Read the model definition and answer for the solid it produces. Units are mm, in the model's axes. Face numbers are marked on the shaded views. A direction names the side the tool comes from. Give positions to 0.01 mm unless a question says otherwise; leave off trailing zeros. Order: outer loops, then holes, each group sorted by start corner. A loop starts at its lowest first (then second) coordinate and runs counter-clockwise, first axis right, second up. Notation, with made-up numbers: (88, -7) - (144, -7) arc R13 ccw to (144, 17) - close; hole circle Ø1 at (3, 22.5). An arc over 180 degrees is marked (long way). One line per item, written item: value. Start each with the question number.
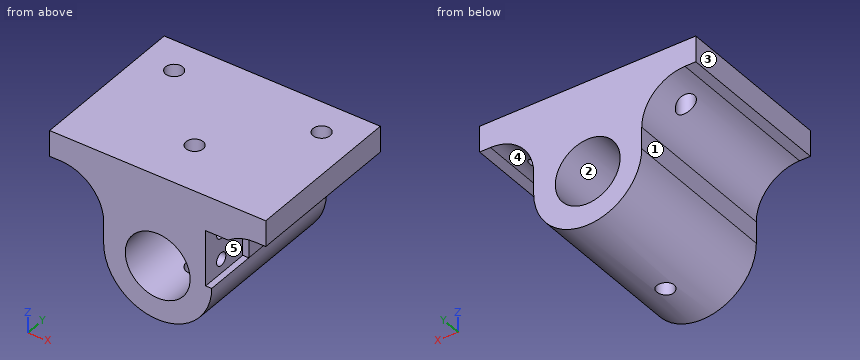
```python
from build123d import *

# Parameters (mm, degrees)
PROFILE_SKETCH1_R                         = 7.5
PROFILE_BOSS_EXTRUDE2_DEPTH               = 37.25987
FASTENINGHOLESKETCH3_R                    = 2
FASTENINGHOLECUT_EXTRUDE8_DEPTH           = 56.995963358
LM8UUFASTENINGHOLESKETCH5_R               = 2
LM8UUFASTENINGHOLECUT_EXTRUDE9_DEPTH      = 56.995963425
MICROSWITCHCUT_EXTRUDE1_DEPTH             = 12.05
MICROSWITCHMOUNTINGHOLESKETCH2_R          = 1.5
MICROSWITCHMOUNTINGHOLECUT_EXTRUDE2_DEPTH = 3.1


with BuildPart() as part:
    # Profile-Sketch1 → Profile-Boss-Extrude2 (new body)
    with BuildSketch(Plane(origin=(0, 0, 0), x_dir=(1, 0, 0), z_dir=(0, 1, 0))):
        with BuildLine():
            Line((-25, -21), (25, -21))
            Line((25, -21), (25, -15))
            Line((25, -15), (22.5, -15))
            ThreePointArc((22.5, -15), (15.428932188, -12.071067812), (12.5, -5))
            Line((12.5, -5), (12.5, 0))
            ThreePointArc((12.5, 0), (0, 12.5), (-12.5, 0))
            Line((-12.5, 0), (-12.5, -5))
            ThreePointArc((-12.5, -5), (-15.428932188, -12.071067812), (-22.5, -15))
            Line((-22.5, -15), (-25, -15))
            Line((-25, -15), (-25, -21))
        make_face()
        with Locations(Location((0, 0, 0), (0, 0, 270))):
            Circle(PROFILE_SKETCH1_R, mode=Mode.SUBTRACT)
    extrude(amount=PROFILE_BOSS_EXTRUDE2_DEPTH)

    # FasteningHoleSketch3 → FasteningHoleCut-Extrude8 (cut, through all)
    with BuildSketch(Plane.XY.offset(21)):
        with Locations((-17.0625, 29.32237)):
            Circle(FASTENINGHOLESKETCH3_R)
        with Locations((17.0625, 29.32237)):
            Circle(FASTENINGHOLESKETCH3_R)
    extrude(amount=-FASTENINGHOLECUT_EXTRUDE8_DEPTH, mode=Mode.SUBTRACT)

    # LM8UUFasteningHoleSketch5 → LM8UUFasteningHoleCut-Extrude9 (cut, through all)
    with BuildSketch(Plane.XY.offset(21)):
        with Locations((0, 12)):
            Circle(LM8UUFASTENINGHOLESKETCH5_R)
    extrude(amount=-LM8UUFASTENINGHOLECUT_EXTRUDE9_DEPTH, mode=Mode.SUBTRACT)

    # Sketch1 → MicroSwitchCut-Extrude1 (cut)
    with BuildSketch(Plane.XZ):
        Polygon((13.9, 12.85), (16.363847734, 12.85), (13.9, 10.102940329), (13.9, 0), (11.1, 0), (11.1, 12.85), align=None)
    extrude(amount=-MICROSWITCHCUT_EXTRUDE1_DEPTH, mode=Mode.SUBTRACT)

    # MicroSwitchMountingHoleSketch2 → MicroSwitchMountingHoleCut-Extrude2 (cut)
    with BuildSketch(Plane(origin=(11.1, 0, 0), x_dir=(0, 0, -1), z_dir=(1, 0, 0))):
        with Locations((-9.6, 5.05)):
            Circle(MICROSWITCHMOUNTINGHOLESKETCH2_R)
        with Locations((-3.25, 5.05)):
            Circle(MICROSWITCHMOUNTINGHOLESKETCH2_R)
    extrude(amount=-MICROSWITCHMOUNTINGHOLECUT_EXTRUDE2_DEPTH, mode=Mode.SUBTRACT)


solid = part.part
```
1) Section B-B on y = 5.05 is taken. Write down the section's boundary in (x, z), plus the area to 3 significant figures.
2) The mould has two halves that part along Z. Classify the marked faces 3, 4 and 5: +Z half, -Z half, draft (parallel to the pull), parting line (faces both ways), or undercut.
3) Section C-C on z = 18 is taken. Write down the section's boundary in (x, y), plus the area to 3 significant figures.
4) For the marked faces 1 and 2, determine the directions among +Z, -Z, +X, -X, +Y, -Y from which every point of the face is accessible in a straight line to the end or side of a thin tool.
5) Section D-D on z = -4 is taken. Write down the section's boundary in (x, y).
6) Find the intervals of material crossed by probe 1 along Y at (x, z) = (10, 9.6); probe 2 along Z at (x, y) = (9, 5); probe 3 along Y at (x, z) = (0, -8), in increasing order. Write a range as from..to.
7) Each of these flat-tipped pins is pushed along its axis until it touches: pin 1 (2.5 mm diameter, centred on x = -17.06, y = 29.32, fed in from -Z); pin 2 (12 mm diameter, centred on x = -17, y = 13.5, fed in from -Z); pin 3 (0.9 mm diameter, centred on y = 5.5, z = 2.5, fed in from +X); pin 4 (9.5 mm diameter, centred on y = 7, z = 8, fed in from +X). Where does it stop, or does it pass through?
8) Section A-A on x = 0 is taken. Write down the section's boundary in (y, z).
Solved:
1. outline: (-25, 15) - (-22.5, 15) arc R10 cw to (-12.5, 5) - (-12.5, 0) arc R12.5 ccw to (12.5, 0) - (11.1, 0) - (11.1, 1.75) - (8, 1.75) - (8, 4.75) - (11.1, 4.75) - (11.1, 8.1) - (8, 8.1) - (8, 11.1) - (11.1, 11.1) - (11.1, 12.85) - (16.31, 12.85) arc R10 cw to (22.5, 15) - (25, 15) - (25, 21) - (-25, 21) - close; hole circle Ø15 at (0, 0)
1. area: 741 mm2
2. face 3: draft
2. face 4: -Z half
2. face 5: undercut
3. outline: (-25, 0) - (25, 0) - (25, 37.26) - (-25, 37.26) - close; hole circle Ø4 at (-17.06, 29.32); hole circle Ø4 at (0, 12); hole circle Ø4 at (17.06, 29.32)
3. area: 1,830 mm2
4. face 1: -Z, -X, +Y, -Y
4. face 2: +Y, -Y
5. outline: (-11.84, 0) - (-6.34, 0) - (-6.34, 37.26) - (-11.84, 37.26) - close; (6.34, 0) - (11.84, 0) - (11.84, 37.26) - (6.34, 37.26) - close
6. probe 1: y = 0..3.55, 6.55..37.26
6. probe 2: z = -8.67..1.75, 4.75..8.1, 11.1..21
6. probe 3: y = 0..10, 14..37.26
7. pin 1: passes through
7. pin 2: stops at z = -5.94
7. pin 3: stops at x = 8
7. pin 4: stops at x = 11.1
8. outline: (0, -12.5) - (10, -12.5) - (10, -7.5) - (0, -7.5) - close; (0, 7.5) - (10, 7.5) - (10, 21) - (0, 21) - close; (14, -12.5) - (37.26, -12.5) - (37.26, -7.5) - (14, -7.5) - close; (14, 7.5) - (37.26, 7.5) - (37.26, 21) - (14, 21) - close
